```python
from build123d import *

# Parameters (mm, degrees)
F1_DEPTH = 63.5
F2_DEPTH = 8.255
F0_W     = 23.3708900283
F0_H     = 19.05
F3_DEPTH = 25.4


with BuildPart() as f1:
    # F0 (on Front) → F1 (new body, symmetric)
    with BuildSketch(Plane.XZ):
        Polygon((26.3337325305, 11.4268229101), (-37.1662674695, 11.4268229101), (-37.1662674695, -7.6231770899), (45.3837325305, -7.6231770899), (45.3837325305, 11.4268229101), align=None)
    extrude(amount=F1_DEPTH, both=True)

    # F0 (on Front) → F2 (join, symmetric)
    with BuildSketch(Plane.XZ):
        with BuildLine():
            add(Edge.make_bspline(
                [(58.6294981139, 63.8270229101), (17.0676354319, 62.8202483058), (-37.0535068214, 41.7246408761), (-37.1662674695, 11.4268229101)],
                knots=[0, 0, 0, 0, 109.1907031929, 109.1907031929, 109.1907031929, 109.1907031929], degree=3))
            Line((-37.1662674695, 11.4268229101), (26.3337325305, 11.4268229101))
            Line((26.3337325305, 11.4268229101), (26.3337325305, 29.0011309419))
            ThreePointArc((26.3337325305, 29.0011309419), (35.6503194891, 52.7490741476), (58.6294981139, 63.8270229101))
        make_face()
    extrude(amount=F2_DEPTH, both=True)

    # F0 (on Front) → F3 (join, symmetric)
    with BuildSketch(Plane.XZ):
        with BuildLine():
            Line((26.3337325305, 29.0011309419), (26.3337325305, 11.4268229101))
            Line((26.3337325305, 11.4268229101), (45.3837325305, 11.4268229101))
            Line((45.3837325305, 11.4268229101), (45.3837325305, 29.0011309419))
            ThreePointArc((45.3837325305, 29.0011309419), (49.4237818094, 39.5817531556), (59.4876149153, 44.7770229101))
            Line((59.4876149153, 44.7770229101), (66.4628425021, 44.7770229101))
            Line((66.4628425021, 44.7770229101), (66.4628425021, 63.8270229101))
            Line((66.4628425021, 63.8270229101), (58.6294981139, 63.8270229101))
            ThreePointArc((58.6294981139, 63.8270229101), (35.6503194891, 52.7490741476), (26.3337325305, 29.0011309419))
        make_face()
        with Locations((78.1482875163, 54.3020229101)):
            Rectangle(F0_W, F0_H)
    extrude(amount=F3_DEPTH, both=True)


solid = f1.part
```
Geometry check sheet. Reference: the model listing, model coordinates, mm. A direction names the side the tool comes from. Coordinates: 2 decimals unless noted, no trailing zeros. Order: outer loops, then holes, each group sorted by start corner. A loop starts at its lowest first (then second) coordinate and runs counter-clockwise, first axis right, second up.
Q1. Tool access check on faces 1 (the face through (51, -25.4, 44)), 2 (the face through (26.334, 17, 20)), 3 (the face through (35.9, -16.948, 53.016)), 4 (the face through (74, 0, 44.777)), 5 (the face through (51, 25.4, 44)). Record the directions out of +Z, -Z, +X, -X, +Y, -Y that give a thin tool (end or side, any length) a straight path to the whole face; none if there is none.
Reply:
face 1: +Z, +X, -X, -Y
face 2: +Z, -X, +Y
face 3: +Z, -X, -Y
face 4: -Z, +X, +Y, -Y
face 5: +Z, +X, -X, +Y
Q2. Sectioned sample at A-A on z = 7. Record the cut outline in (x, y), and give its area (3 significant figures).
Reply:
outline: (-37.17, -63.5) - (45.38, -63.5) - (45.38, 63.5) - (-37.17, 63.5) - close
area: 10,500 mm2
Q3. Sectioned sample at B-B on y = -35.5. Record the cut outline in (x, z), and give its area (3 significant figures).
Reply:
outline: (-37.17, -7.62) - (45.38, -7.62) - (45.38, 11.43) - (-37.17, 11.43) - close
area: 1,570 mm2
Q4. Depth check by flat-ended pin: pin 1 Ø12 at (x, z) = (60, 39.5) entering from +Y; pin 2 Ø13.5 at (y, z) = (-14, 22) entering from -X; pin 3 Ø18.5 at (y, z) = (16.5, 5.5) entering from +X; pin 4 Ø12 at (x, z) = (53.5, 3) entering from -Y. Enter the tip coordinate at first touch or a pass-through.
Reply:
pin 1: stops at y = 25.4
pin 2: stops at x = -36.15
pin 3: stops at x = 45.38
pin 4: passes through
Q5. Thickness scan on probe 1 along Z at (x, y) = (-17.5, -35.5); probe 2 along Y at (x, z) = (20, 48.5) (3 decimals); probe 3 along Y at (x, z) = (81, 61). Record the ranges inside material, lowest first.
Reply:
probe 1: z = -7.62 to 11.43
probe 2: y = -8.255 to 8.255
probe 3: y = -25.4 to 25.4
